Check sheet for the modelled part. Datum: model origin and axes. Units: mm. A direction names the side the tool comes from. Give positions to 0.01 mm unless a question says otherwise; leave off trailing zeros. Write each loop counter-clockwise with the first axis right and the second up, starting at its lowest first coordinate (ties: lowest second). Pieces come first, ordered by that corner, then holes. Notation, with made-up numbers: (-39, -12) -> (4, -12) arc R7 ccw to (4, -5) -> close; hole circle Ø10 at (-10, -8.75). An arc over 180 degrees is marked (long way). Return JSON: item names as keys, results as strings.
from build123d import *

# Parameters (mm, degrees)
SKETCH1_W           = 22.5
SKETCH1_H           = 202
BOSS_EXTRUDE1_DEPTH = 20
SKETCH2_W           = 22.5
SKETCH2_H           = 18
CUT_EXTRUDE1_DEPTH  = 2
CHAMFER5_SIZE       = 2.060608065
CHAMFER5_SIZE_2     = 0.75
FILLET5_R           = 0.4
SKETCH3_W           = 60
SKETCH3_H           = 2.5
CUT_EXTRUDE2_DEPTH  = 22.5


with BuildPart() as part:
    # Sketch1 → Boss-Extrude1 (new body)
    with BuildSketch(Plane(origin=(0, 0, 0), x_dir=(0, 1, 0), z_dir=(0, 0, 1))):
        with Locations((11.25, -101)):
            Rectangle(SKETCH1_W, SKETCH1_H)
    extrude(amount=-BOSS_EXTRUDE1_DEPTH)

    # Sketch2 → Cut-Extrude1 (cut)
    with BuildSketch(Plane.YZ.offset(202)):
        with Locations((11.25, -11)):
            Rectangle(SKETCH2_W, SKETCH2_H)
    extrude(amount=-CUT_EXTRUDE1_DEPTH, mode=Mode.SUBTRACT)

    # Chamfer5
    # the kernel refuses this chamfer: 2.060608065, 0.75 mm, written as the material it takes off along each edge
    with BuildSketch(Plane(origin=(202, 27.845618587, -2), x_dir=(-0.9999130865277316, 0, -0.013184058198645886), z_dir=(0, -1, 0))) as chamfer5_piece_1_section:
        Polygon((CHAMFER5_SIZE * 0.999913086329, -CHAMFER5_SIZE * 0.013184058196), (-CHAMFER5_SIZE_2 * 0.0131840581986, -CHAMFER5_SIZE_2 * 0.999913086528), (0, 0), align=None)
    chamfer5_piece_1 = extrude(amount=33.191237174, mode=Mode.PRIVATE)
    chamfer5_piece_1 = split(chamfer5_piece_1, bisect_by=Plane(origin=(200, 11.25, -1.766801206), z_dir=(1, 0, 0)), keep=Keep.TOP, mode=Mode.PRIVATE)
    add(chamfer5_piece_1, mode=Mode.SUBTRACT)

    # Fillet5
    fillet5_edges = [part.edges().sort_by_distance(p)[0] for p in [
        (202, 0, -0.625),
        (202, 22.5, -0.625),
    ]]
    fillet(fillet5_edges, radius=FILLET5_R)

    # Sketch3 → Cut-Extrude2 (cut)
    with BuildSketch(Plane(origin=(0, 22.5, 0), x_dir=(-1, 0, 0), z_dir=(0, 1, 0))):
        with Locations((-30, -1.25)):
            Rectangle(SKETCH3_W, SKETCH3_H)
    extrude(amount=-CUT_EXTRUDE2_DEPTH, mode=Mode.SUBTRACT)


solid = part.part
(1) Thickness scan on L1, parallel to X at y = 13, z = -9.5; L2, parallel to Z at x = 58.5, y = 14. Record the ranges inside material, lowest first.
Reply:
{"L1": "0 to 200", "L2": "-20 to -2.5"}
(2) Cross-section at B-B on x = 28. Enter the section's corners in (y, z), then the cut area to 3 significant figures.
Reply:
{"outline": "(0, -20) -> (22.5, -20) -> (22.5, -2.5) -> (0, -2.5) -> close", "area": "394 mm^2"}
(3) Set-up check for faces 1 (the flat face through (200, 11, -11)), 2 (the flat face through (102, 0, -10)), 3 (the flat face through (30, 11, -2.5)): record each of +Z, -Z, +X, -X, +Y, -Y from which the full face is reachable in a straight line by a thin tool's end or side.
Reply:
{"face 1": "-Z, +X, +Y, -Y", "face 2": "+Z, -Z, +X, -X, -Y", "face 3": "+Z, -X, +Y, -Y"}
(4) Cross-section at A-A on y = 11.25. Enter the section's corners in (x, z), then the cut area to 3 significant figures.
Reply:
{"outline": "(0, -20) -> (200, -20) -> (200, -1.98) -> (202, -1.25) -> (202, 0) -> (60, 0) -> (60, -2.5) -> (0, -2.5) -> close", "area": "3,850 mm^2"}
(5) Depth check by flat-ended pin: pin 1 Ø7 at (x, y) = (27, 6) entering from +Z; pin 2 Ø3 at (y, z) = (5.5, -10) entering from +X; pin 3 Ø5 at (y, z) = (10, -3) entering from +X; pin 4 Ø2 at (y, z) = (16.5, -1) entering from -X. Enter the tip coordinate at first touch or a pass-through.
Reply:
{"pin 1": "z = -2.5", "pin 2": "x = 200", "pin 3": "x = 202", "pin 4": "x = 60"}
